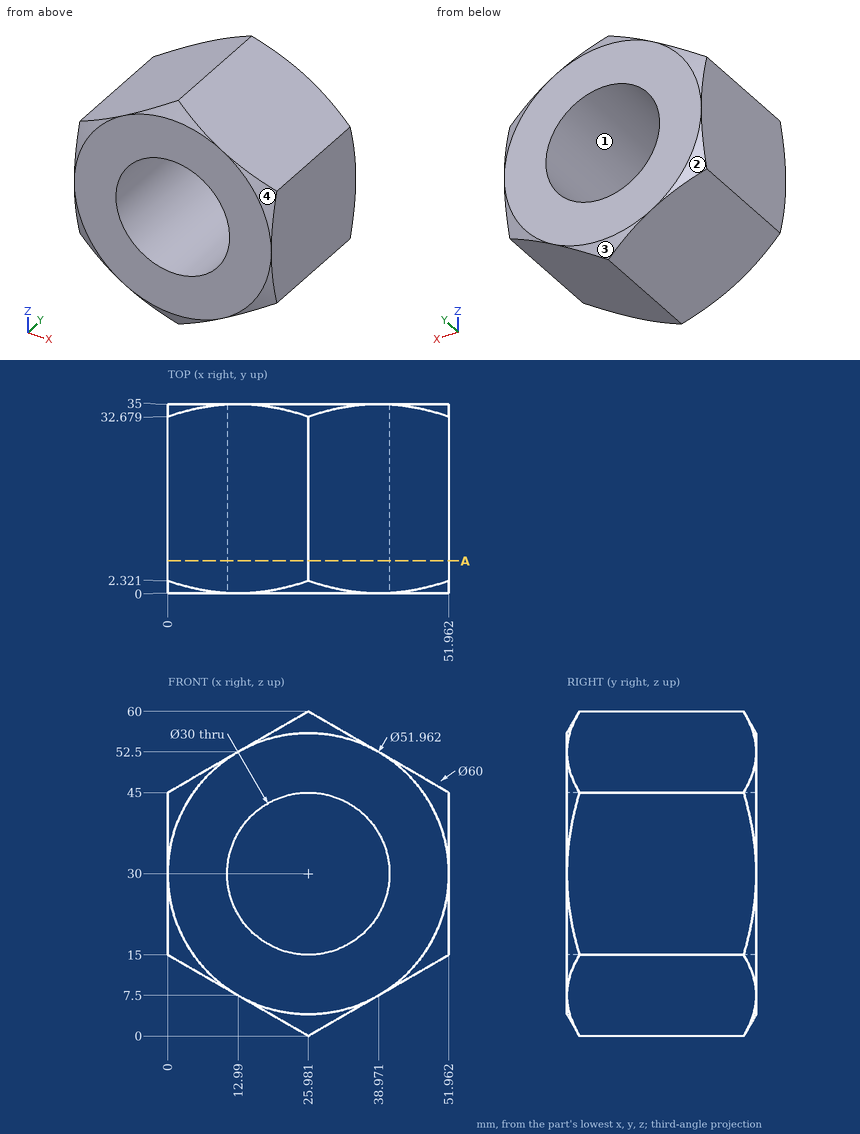
Geometry check sheet. Reference: drawing and pictorial views, mm from the part's lowest x, y, z. Coordinates: 2 decimals unless noted, no trailing zeros. Order: outer loops, then holes, each group sorted by start corner. A loop starts at its lowest first (then second) coordinate and runs counter-clockwise, first axis right, second up.
1. Release check for a two-part mould opening along X. For the marked faces 1, 2, 3 and 4 record: +X half, -X half, draft (parallel to the pull), parting line (faces both ways), or undercut.
Results found:
face 1: undercut
face 2: -X half
face 3: parting line
face 4: +X half
2. Scan lines: line 1 (Z direction, x = 26, y = 17.5); line 2 (Z direction, x = 32, y = 6.5) (1 decimal); line 3 (X direction, y = 11, z = 28) (1 decimal). Record each from-to range of solid material in increasing order.
Results found:
line 1: z = 0.01 to 15, 45 to 59.99
line 2: z = 3.5 to 16.3, 43.7 to 56.5
line 3: x = 0 to 11.1, 40.8 to 52
3. Go/stop test with flat-tipped pins: pin 1 Ø6 at (x, y) = (30.5, 5) entering from +Z; pin 2 Ø5 at (x, y) = (34, 6.5) entering from +Z; pin 3 Ø24 at (x, z) = (25.98, 30) entering from +Y; pin 4 Ø4 at (x, y) = (39, 9.5) entering from -Z. Record where each tip stops, or that it passes through.
Results found:
pin 1: stops at z = 59.12
pin 2: stops at z = 56.81
pin 3: passes through
pin 4: stops at z = 6.36
4. Sectioned sample at A-A, the plane y = 6. Record the cut outline in (x, z), and give its area (3 significant figures).
Results found:
outline: (0, 15) - (25.98, 0) - (51.96, 15) - (51.96, 45) - (25.98, 60) - (0, 45) - close; hole circle Ø30 at (25.98, 30)
area: 1,630 mm2
